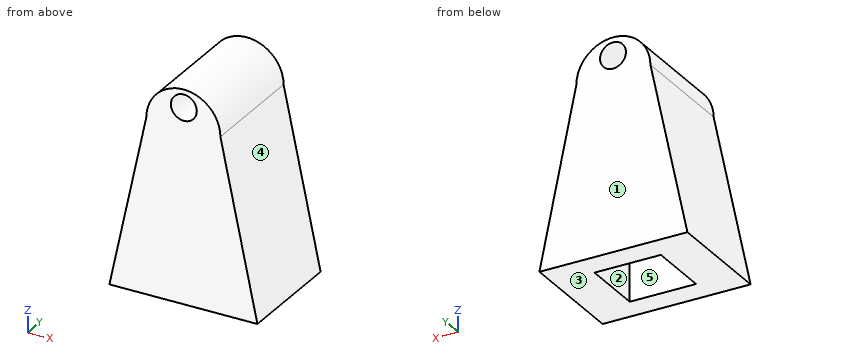
```python
from build123d import *

# Parameters (mm, degrees)
F1_DEPTH = 30
F2_W     = 17.9273141921
F2_H     = 16.7198758554
F3_DEPTH = 47.8
F5_D     = 7


with BuildPart() as f1:
    # F0 (on Front) → F1 (new body)
    with BuildSketch(Plane.XZ):
        Polygon((10, 47.186203301), (0, 0), (40, 0), (30, 47.186203301), (20, 47.186203301), align=None)
        with BuildLine():
            ThreePointArc((30, 47.186203301), (20, 57.1520274516), (10, 47.186203301))
            Line((10, 47.186203301), (20, 47.186203301))
            Line((20, 47.186203301), (30, 47.186203301))
        make_face()
    extrude(amount=F1_DEPTH)

    # F2 (on Top) → F3 (cut, symmetric)
    with BuildSketch(Plane.XY):
        with Locations((20, -15.1315899557)):
            Rectangle(F2_W, F2_H)
    extrude(amount=F3_DEPTH, both=True, mode=Mode.SUBTRACT)

    # F5 (through all)
    with Locations(Plane(origin=(0, 0, 0), x_dir=(-1, 0, 0), z_dir=(0, 1, 0))):
        with Locations((-20.1143659651, 52.3227863014)):
            Hole(F5_D / 2)


solid = f1.part
```
Build history of the part. All positions in model axes, mm. Face numbers are marked on the shaded views. A direction names the side the tool comes from. Coordinates: 2 decimals unless noted, no trailing zeros. Write each loop counter-clockwise with the first axis right and the second up, starting at its lowest first coordinate (ties: lowest second). Pieces come first, ordered by that corner, then holes.
1. Drop flat-ended pins along their axis: pin 1 (10 mm diameter, centred on y = -6, z = 35.5, fed in from -X); pin 2 (6 mm diameter, centred on x = 13.5, y = -26.5, fed in from -Z); pin 3 (3 mm diameter, centred on y = -15, z = 42, fed in from -X); pin 4 (5 mm diameter, centred on x = 28, y = -16, fed in from +Z). Give the stop position or say it passes through.
Answer block:
pin 1: stops at x = 6.46
pin 2: stops at z = 0
pin 3: stops at x = 8.58
pin 4: stops at z = 55.5
2. Band-saw the part on A-A, the plane x = 20. Give the cut face in (y, z).
Answer block:
outline: (-30, 0) - (-23.49, 0) - (-23.49, 47.8) - (-6.77, 47.8) - (-6.77, 0) - (0, 0) - (0, 48.82) - (-30, 48.82) - close; (-30, 55.82) - (0, 55.82) - (0, 57.15) - (-30, 57.15) - close
3. Band-saw the part on B-B, the plane z = 39.5. Give the cut face in (x, y).
Answer block:
outline: (8.37, -30) - (31.63, -30) - (31.63, 0) - (8.37, 0) - close; hole (11.04, -23.49) - (28.96, -23.49) - (28.96, -6.77) - (11.04, -6.77) - close
4. 3-axis set-ups, long thin cutter, end or side, ignore diameter. For the marked faces 1 and 2: which of +Z, -Z, +X, -X, +Y, -Y reach the whole face in a straight line?
Answer block:
face 1: +Z, -Z, +X, -X, +Y
face 2: -Z
5. Band-saw the part on C-C, the plane y = -15. Give the cut face in (x, z).
Answer block:
outline: (0, 0) - (11.04, 0) - (11.04, 47.8) - (28.96, 47.8) - (28.96, 0) - (40, 0) - (30, 47.19) arc R10 ccw to (10, 47.19) - close; hole circle Ø7 at (20.11, 52.32)
6. Band-saw the part on D-D, the plane z = 53.5. Give the cut face in (x, y), and give its area (3 significant figures).
Answer block:
outline: (12.27, -30) - (16.82, -30) - (16.82, 0) - (12.27, 0) - close; (23.41, -30) - (27.73, -30) - (27.73, 0) - (23.41, 0) - close
area: 266 mm2
7. Pull direction X, two halves, no side cores. Call the marked faces 3, 4 and 5: released by +X, released by -X, zero draft, split by the parting line, or undercut.
Answer block:
face 3: zero draft
face 4: released by +X
face 5: undercut
8. Drill centre lines: probe 1 along Y at (x, z) = (23.5, 12); probe 2 along Z at (x, y) = (20, -8.5); probe 3 along X at (y, z) = (-18.5, 20). Where is each one in solid material? Low to high.
Answer block:
probe 1: y = -30 to -23.49, -6.77 to 0
probe 2: z = 47.8 to 48.82, 55.82 to 57.15
probe 3: x = 4.24 to 11.04, 28.96 to 35.76
